Autodesk Inventor part; units mm, degrees
ref_plane "YZ Plane" through (0, 0, 0) normal (1, 0, 0) x (0, 1, 0)
ref_plane "XZ Plane" through (0, 0, 0) normal (0, 1, 0) x (-1, 0, 0)
ref_plane "XY Plane" through (0, 0, 0) normal (0, 0, 1) x (1, 0, 0)
sketch "Sketch1" plane through (0, 0, 0) normal (0, 1, 0) x (-1, 0, 0)
  line L0 (-1.1714, -12.4618) -> (-1.1714, -27.4618) construction
  line L1 (8.1, -25.7) -> (8.1, -10.7) construction
  line L2 (-1.1714, -21.2152) -> (8.1, -21.2152) construction
  line L3 (3.4643, -21.2152) -> (3.4643, 9.1343) construction
  line L4 (-3.267, -19.9618) -> (-1.0357, -19.9618)
  line L5 (-1.0357, -19.9618) -> (-1.0357, -13.9618)
  line L6 (-1.0357, -13.9618) -> (-3.267, -13.9618)
  line L7 (-4.2857, -14.3912) -> (-4.2857, -19.5563)
  arc A0 (-4.2857, -19.5563) -> (-3.267, -19.9618) centre (-3.267, -18.4795) ccw
  arc A1 (-3.267, -13.9618) -> (-4.2857, -14.3912) centre (-3.267, -15.3848) ccw
  point P0 (0, 0)
  dimension "d0" = 7.75
  dimension "d1" = 4.5
  dimension "d2" = 6
revolve "Revolution1" add sketch "Sketch1" angle 360 about axis through (-3.4643, 0, -21.2152) along (0, 0, 1)
sketch "Sketch2" plane through (-3.4643, 0, -13.9618) normal (0, 0, 1) x (1, 0, 0)
  circle A0 centre (0.0167, -8.8653) radius 1.75
  circle A1 centre (6.2805, -6.2569) radius 1.75
  circle A2 centre (8.8653, 0.0167) radius 1.75
  circle A3 centre (6.2569, 6.2805) radius 1.75
  circle A4 centre (-0.0167, 8.8653) radius 1.75
  circle A5 centre (-6.2805, 6.2569) radius 1.75
  circle A6 centre (-8.8653, -0.0167) radius 1.75
  circle A7 centre (-6.2569, -6.2805) radius 1.75
  point P0 (3.4643, 0)
  point P1 (0, 0)
  dimension "d4" = 3.5
  dimension "d7" = 360
extrude "Extrusion1" cut sketch "Sketch2" against normal blind 10 contours A0 | A1 | A3 | A4 | A5 | A6 | A7
sketch "Sketch3" plane through (-3.4643, 0, -13.9618) normal (0, 0, 1) x (1, 0, 0)
  line L0 (0, 0) -> (8.4123, 0) construction
  line L1 (8.4123, 0) -> (8.4123, -1.25)
  line L2 (8.4123, -1.25) -> (0, -1.25)
  line L3 (0, -1.25) -> (0, 0)
  line L4 (8.4123, 0) -> (8.4123, 1.25)
  line L5 (8.4123, 1.25) -> (0, 1.25)
  line L6 (0, 1.25) -> (0, 0)
  point P0 (3.4643, 0)
  dimension "d11" = 1.25
extrude "Extrusion2" cut sketch "Sketch3" against normal blind 10
properties part number "PWTR-0108" material "Aluminum 6061"
Source: CAD feature listing. Evaluate the final solid. Frame: model axes, mm. A direction names the side the tool comes from. Coordinates: 2 decimals unless noted, no trailing zeros. Order: outer loops, then holes, each group sorted by start corner. A loop starts at its lowest first (then second) coordinate and runs counter-clockwise, first axis right, second up. Notation, with made-up numbers: M 48.5,17.5 L 93.5,17.5 A6 cw 93.5,28.5 Z; hole C 13.5,32.25 d6. An arc over 180 degrees is marked long. Write each question's results on one line, items separated by ' | '. Start each with the question number.
1) Contact query for flat-ended pins moving along their axis: pin 1 Ø3.5 at (x, z) = (2.5, -15.5) entering from -Y; pin 2 Ø1.5 at (x, z) = (-6, -16) entering from +Y; pin 3 Ø2 at (x, z) = (-2, -17.5) entering from -Y. Output: stop coordinate, or through.
2) Draft query along X for faces 3 (the face through (-3.431, -7.115, -16.922)), 4 (the face through (3, 1.25, -17)), 5 (the face through (-0.535, 7.175, -17.01)). Return one class per face: released by +X, released by -X, zero draft, split by the parting line, or undercut.
3) Access query for faces 1 (the face through (-4, 5, -19.962)), 2 (the face through (3, -1.25, -17)). Directions: +Z, -Z, +X, -X, +Y, -Y. A direction counts if a zero-diameter tool reaches every point of the face in a straight line with its end or side. Return the directions, or none.
4) Line query: line 1 (X direction, y = 0, z = -15.25); line 2 (Y direction, x = -6.75, z = -17.5); line 3 (Y direction, x = -1, z = -14.25). Output: solid intervals per line, ascending. Write a range as from..to.
5) Section query A-A (z = -14.75). Return the cut outline in (x, y).
Answers:
1) pin 1: stops at y = -6.5 | pin 2: stops at y = 7.54 | pin 3: stops at y = -7.65
2) face 3: undercut | face 4: zero draft | face 5: released by +X
3) face 1: -Z, +X, -X, +Y, -Y | face 2: +Z, -Z, +X
4) line 1: x = -10.58..-7.96 | line 2: y = -7.02..-3.07, 3.07..7.02 | line 3: y = -7.18..-3.77, 3.77..7.18
5) outline: M -11.11,-1.27 A7.75 ccw -9.75,-4.53 A1.75 cw -7.97,-6.3 A7.75 ccw -4.71,-7.65 A1.75 cw -2.19,-7.65 A7.75 ccw 1.07,-6.29 A1.75 cw 2.84,-4.51 A7.75 ccw 4.18,-1.25 L 0.86,-1.25 A4.5 cw long 0.86,1.25 L 4.18,1.25 A7.75 ccw 2.82,4.53 A1.75 cw 1.04,6.3 A7.75 ccw -2.22,7.65 A1.75 cw -4.74,7.65 A7.75 ccw -8,6.29 A1.75 cw -9.77,4.51 A7.75 ccw -11.11,1.24 A1.75 cw Z
